from build123d import *

# Parameters (mm, degrees)
CROQUIS1_R              = 1.143
SALIENTE_EXTRUIR6_DEPTH = 1.5875


with BuildPart() as part:
    # Croquis1 → Saliente-Extruir6 (new body)
    with BuildSketch(Plane(origin=(0, 0, 0), x_dir=(1, 0, 0), z_dir=(0, 1, 0))):
        with BuildLine():
            ThreePointArc((-13.782319099, 2.794), (-16.576319099, 0), (-13.782319099, -2.794))
            add(Edge.make_bspline(
                [(-13.782319099, -2.794), (-12.381959509, -2.745210856), (-11.808442523, -3.043224941), (-9.906232869, -4.4207888)],
                knots=[0, 0, 0, 0, 1, 1, 1, 1], degree=3))
            ThreePointArc((-9.906232869, -4.4207888), (-7.051319099, -5.2625), (-4.196405329, -4.4207888))
            add(Edge.make_bspline(
                [(-4.196405329, -4.4207888), (-2.294195675, -3.043224941), (-1.720678689, -2.745210856), (-0.320319099, -2.794)],
                knots=[0.921934519, 0.921934519, 0.921934519, 0.921934519, 1.921934519, 1.921934519, 1.921934519, 1.921934519], degree=3))
            ThreePointArc((-0.320319099, -2.794), (2.473680901, 0), (-0.320319099, 2.794))
            add(Edge.make_bspline(
                [(-0.320319099, 2.794), (-1.720678689, 2.745210856), (-2.294195675, 3.043224941), (-4.196405329, 4.4207888)],
                knots=[0, 0, 0, 0, 1, 1, 1, 1], degree=3))
            ThreePointArc((-4.196405329, 4.4207888), (-7.051319099, 5.2625), (-9.906232869, 4.4207888))
            add(Edge.make_bspline(
                [(-9.906232869, 4.4207888), (-11.808442523, 3.043224941), (-12.381959509, 2.745210856), (-13.782319099, 2.794)],
                knots=[0.921934519, 0.921934519, 0.921934519, 0.921934519, 1.921934519, 1.921934519, 1.921934519, 1.921934519], degree=3))
        make_face()
        with Locations((-13.782319099, 0)):
            Circle(CROQUIS1_R, mode=Mode.SUBTRACT)
        with Locations((-0.320319099, 0)):
            Circle(CROQUIS1_R, mode=Mode.SUBTRACT)
    extrude(amount=SALIENTE_EXTRUIR6_DEPTH)


solid = part.part
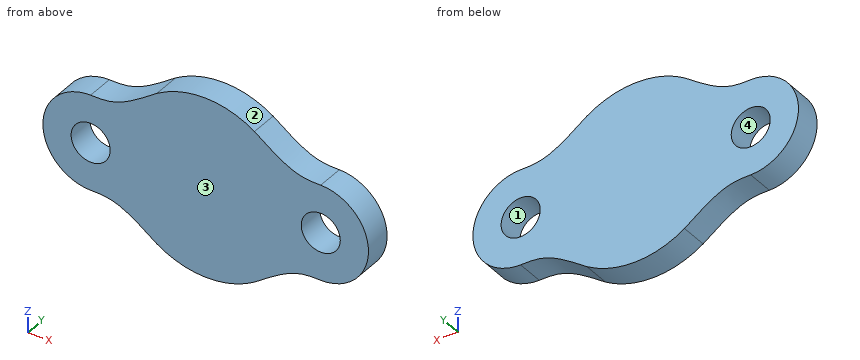
Design review of the part built by this model. Coordinates are the model's own, in mm. Face numbers are marked on the shaded views. Give positions to 0.01 mm unless a question says otherwise; leave off trailing zeros. Order: outer loops, then holes, each group sorted by start corner. A loop starts at its lowest first (then second) coordinate and runs counter-clockwise, first axis right, second up. Notation, with made-up numbers: (-3, 21) - (28, 21) arc R21 ccw to (28, 54) - close; hole circle Ø4 at (70, 86.5). An arc over 180 degrees is marked (long way). Write item = value, one per line. Start each with the question number.
Q1. We need section D-D on z = 2.5. State the section outline as (x, y) points, plus the area to 3 significant figures.
Q2. Clearance check with a flat-ended pin moving along its axis: pin 1 Ø1.4 at (x, z) = (-0.32, 0) entering from +Y. State where the tip first meets the part, or that it passes through.
Q3. We need section B-B on y = 0.95. State how many separate pieces and enclosed holes the cut face has, plus the area to 3 significant figures.
Q4. Mouldability with a two-part tool opening along X and no side actions: class the marked faces 1, 2, 3 and 4 as released by +X, released by -X, zero draft, split by the parting line, or undercut.
Q5. We need section A-A on z = -0.5. State the section outline as (x, y) points.
Q6. To check wall thickness, follow L1, parallel to X at y = 0.55, z = 0; L2, parallel to X at y = 0.8, z = -0.25 (3 decimals); L3, parallel to Z at x = -13, y = 0.8. State the ranges of each line that lie inside material, in increasing order. Write a range as from..to.
Q7. We need section C-C on x = -5.5. State the section outline as (y, z) points, plus the area to 3 significant figures.
Working result:
q1.outline = (-15.03, 0) - (0.93, 0) - (0.93, 1.59) - (-15.03, 1.59) - close
q1.area = 25.3 mm²
q2.pin_1 = through
q3.separate_pieces = 1
q3.enclosed_holes = 2
q3.area = 125 mm²
q4.face_1 = undercut
q4.face_2 = split by the parting line
q4.face_3 = zero draft
q4.face_4 = undercut
q5.outline = (-16.53, 0) - (-14.81, 0) - (-14.81, 1.59) - (-16.53, 1.59) - close; (-12.75, 0) - (-1.35, 0) - (-1.35, 1.59) - (-12.75, 1.59) - close; (0.71, 0) - (2.43, 0) - (2.43, 1.59) - (0.71, 1.59) - close
q6.L1 = -16.58..-14.93, -12.64..-1.46, 0.82..2.47
q6.L2 = -16.565..-14.898, -12.667..-1.436, 0.795..2.462
q6.L3 = -2.81..-0.83, 0.83..2.81
q7.outline = (0, -5.03) - (1.59, -5.03) - (1.59, 5.03) - (0, 5.03) - close
q7.area = 16.0 mm²
